from build123d import *

# Parameters (mm, degrees)
F1_R     = 45.35
F2_DEPTH = 3
F4_R     = 1


with BuildPart() as f2:
    # F1 (on Top) → F2 (new body, symmetric)
    with BuildSketch(Plane.XY):
        Circle(F1_R)
        with BuildLine():
            ThreePointArc((39.3418678526, 0.7999586665), (39.3479669106, 0.4), (39.35, 0))
            ThreePointArc((39.35, 0), (39.3479669106, -0.4), (39.3418678526, -0.7999586665))
            ThreePointArc((39.3418678526, -0.7999586665), (-39.35, 0), (39.3418678526, 0.7999586665))
        make_face(mode=Mode.SUBTRACT)
        with BuildLine():
            ThreePointArc((39.3418678526, -0.7999586665), (39.3479669106, -0.4), (39.35, 0))
            ThreePointArc((39.35, 0), (39.3479669106, 0.4), (39.3418678526, 0.7999586665))
            ThreePointArc((39.3418678526, 0.7999586665), (38.55, 0), (39.3418678526, -0.7999586665))
        make_face()
    extrude(amount=F2_DEPTH, both=True)

    # F4
    f4_edges = [f2.edges().sort_by_distance(p)[0] for p in [
        (-45.35, 0, 3),
        (-45.35, 0, -3),
    ]]
    fillet(f4_edges, radius=F4_R)


solid = f2.part
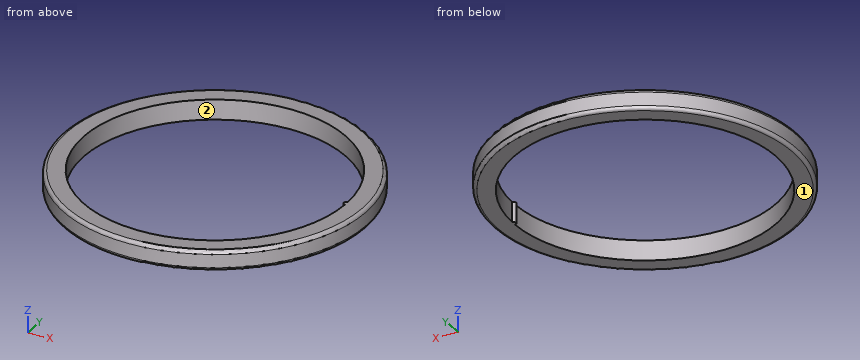
For this review, take the finished solid that the model builds, in its own axes (mm). Face numbers are marked on the shaded views. Coordinates: 2 decimals unless noted, no trailing zeros. Write each loop counter-clockwise with the first axis right and the second up, starting at its lowest first coordinate (ties: lowest second). Pieces come first, ordered by that corner, then holes. Notation, with made-up numbers: (53.5, 51.5) -> (99.5, 51.5) arc R35 cw to (99.5, 83.5) -> close; hole circle Ø4 at (47, 13). An arc over 180 degrees is marked (long way). Write each question's results on one line, items separated by ' | '. Start each with the question number.
1) Consider section A-A (x = 0). Write out the cut boundary in (y, z).
2) Consider section B-B (z = 0.2). Write out the cut boundary in (x, y).
3) Insertion check: pin 1 (2 mm diameter, centred on x = -18.5, z = -2, fed in from +Y); pin 2 (1 mm diameter, centred on x = -1.5, z = 2, fed in from +Y); pin 3 (1 mm diameter, centred on y = -17, z = 2, fed in from +X). Each pin has a flat end and moves straight along its axis. Give the tip position at first contact, or say it passes through.
4) The part is to be moulded in two halves that separate along Y. For the marked faces 1 and 2, say which applies: +Y half, -Y half, draft (parallel to the pull), parting line (faces both ways), or undercut.
5) Wall thickness on L1, parallel to Y at x = 0, z = 0.25; L2, parallel to Y at x = -35, z = -0.8; L3, parallel to X at y = 32.5, z = 2.4: over which ranges is each line inside the solid? List them lowest first. Write a range as [from, to].
Geometry says:
1) outline: (-45.35, -2) arc R1 ccw to (-44.35, -3) -> (-39.35, -3) -> (-39.35, 3) -> (-44.35, 3) arc R1 ccw to (-45.35, 2) -> close; (39.35, -3) -> (44.35, -3) arc R1 ccw to (45.35, -2) -> (45.35, 2) arc R1 ccw to (44.35, 3) -> (39.35, 3) -> close
2) outline: circle Ø90.7 at (0, 0); hole (39.34, -0.8) arc R0.8 cw to (39.34, 0.8) arc R39.35 ccw (long way) to start
3) pin 1: y = 41.84 | pin 2: y = 45.34 | pin 3: x = 42.24
4) face 1: draft | face 2: undercut
5) L1: [-45.35, -39.35], [39.35, 45.35] | L2: [-28.84, -17.98], [17.98, 28.84] | L3: [-31.51, -22.18], [22.18, 31.51]
